The figure shows three views and two pictorial views of one solid part (mm, origin at its lowest corner). Answer the questions. A direction names the side the tool comes from. Coordinates: 2 decimals unless noted, no trailing zeros. Loops run counter-clockwise (first coordinate to the right, second up) from the corner with the lowest first, then second, coordinate; pieces in that order, holes last. Notation, with made-up numbers: M -16,60.25 L -6,60.25 A18 cw -6,88.25 Z; hole C 77.5,4 d11. An arc over 180 degrees is marked long. Answer in a Markdown table with one row per item. Add a question column.
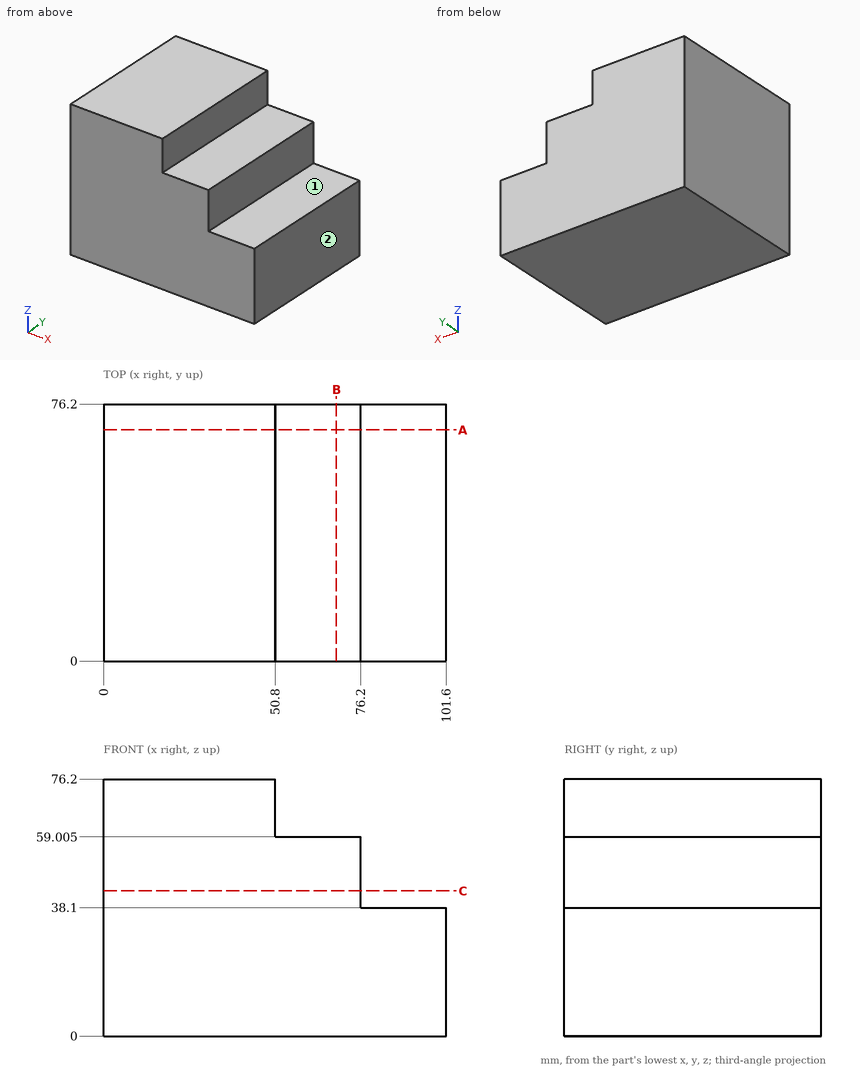
(1) A cutting plane is placed at B-B (x = 69). Give the vertices of the cut face in (y, z) (3 decimals), plus the area to 3 significant figures.
(2) A cutting plane is placed at C-C (z = 43). Give the vertices of the cut face in (x, y).
(3) Each of these flat-tipped pins is pushed along its axis until it touches: pin 1 (12 mm diameter, centred on x = 80, y = 55, fed in from +Z) (3 decimals); pin 2 (14 mm diameter, centred on y = 32, z = 65.5, fed in from +X); pin 3 (12.5 mm diameter, centred on x = 91, y = 32, fed in from +Z). Where does it stop, or does it pass through?
(4) Straight lines are drawn through the part: line 1 (Z direction, x = 88, y = 55); line 2 (X direction, y = 67.5, z = 70.5); line 3 (Z direction, x = 69, y = 18.5) (3 decimals). For each, find the intervals that lie inside material, in ascending order.
(5) A cutting plane is placed at A-A (y = 68.5). Give the vertices of the cut face in (x, z) (3 decimals), plus the area to 3 significant figures.
(6) For the marked faces 1 and 2, determine the directions among +Z, -Z, +X, -X, +Y, -Y from which every point of the face is accessible in a straight line to the end or side of a thin tool.
Solved:
| question | item | result |
|---|---|---|
| 1 | outline | M 0,0 L 76.2,0 L 76.2,59.005 L 0,59.005 Z |
| 1 | area | 4,500 mm² |
| 2 | outline | M 0,0 L 76.2,0 L 76.2,76.2 L 0,76.2 Z |
| 3 | pin 1 | stops at z = 59.005 |
| 3 | pin 2 | stops at x = 76.2 |
| 3 | pin 3 | stops at z = 38.1 |
| 4 | line 1 | z = 0 to 38.1 |
| 4 | line 2 | x = 0 to 50.8 |
| 4 | line 3 | z = 0 to 59.005 |
| 5 | outline | M 0,0 L 101.6,0 L 101.6,38.1 L 76.2,38.1 L 76.2,59.005 L 50.8,59.005 L 50.8,76.2 L 0,76.2 Z |
| 5 | area | 6,340 mm² |
| 6 | face 1 | +Z, +X, +Y, -Y |
| 6 | face 2 | +Z, -Z, +X, +Y, -Y |
